Drawing for the job (mm, zero at the part's lowest x, y, z). Give positions to 0.01 mm unless a question says otherwise; leave off trailing zeros. Write each loop counter-clockwise with the first axis right and the second up, starting at its lowest first coordinate (ties: lowest second). Pieces come first, ordered by that corner, then holes.
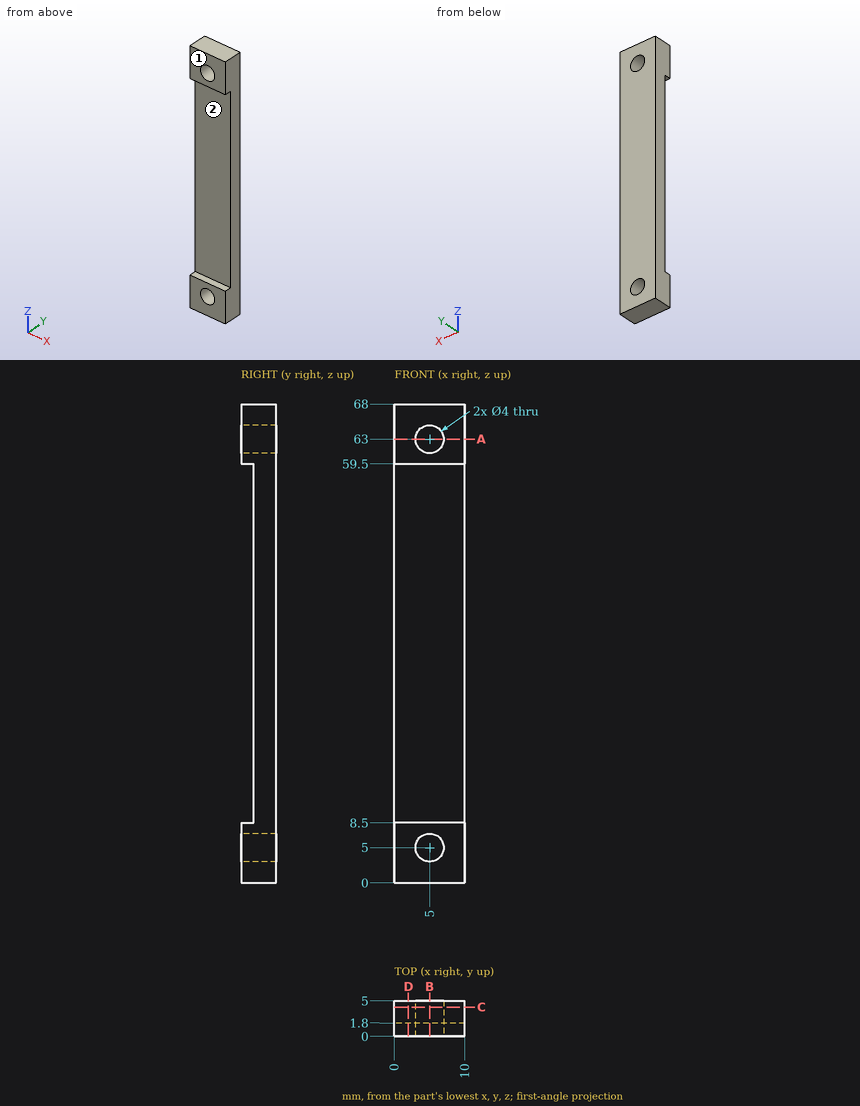
1. Pull direction Z, two halves, no side cores. Call the marked faces 1 and 2: +Z half, -Z half, draft (parallel to the pull), parting line (faces both ways), or undercut.
Calculated:
face 1: draft
face 2: undercut
2. Probe probe 1 along Z at (x, y) = (5, 1.4); probe 2 along Z at (x, y) = (8, 0.2); probe 3 along Z at (x, y) = (5.5, 3.75). List the from-to ranges inside material, lowest first.
Calculated:
probe 1: z = 0 to 3, 7 to 8.5, 59.5 to 61, 65 to 68
probe 2: z = 0 to 8.5, 59.5 to 68
probe 3: z = 0 to 3.06, 6.94 to 61.06, 64.94 to 68
3. Slice it at C-C, the plane y = 4.1. Write the cut outline in (x, z), and give its area (3 significant figures).
Calculated:
outline: (0, 0) - (10, 0) - (10, 68) - (0, 68) - close; hole circle Ø4 at (5, 5); hole circle Ø4 at (5, 63)
area: 655 mm2
4. Slice it at B-B, the plane x = 5. Write the cut outline in (y, z), and give its area (3 significant figures).
Calculated:
outline: (0, 0) - (5, 0) - (5, 3) - (0, 3) - close; (0, 7) - (5, 7) - (5, 61) - (0, 61) - (0, 59.5) - (1.8, 59.5) - (1.8, 8.5) - (0, 8.5) - close; (0, 65) - (5, 65) - (5, 68) - (0, 68) - close
area: 208 mm2
5. Slice it at D-D, the plane x = 2. Write the cut outline in (y, z), and give its area (3 significant figures).
Calculated:
outline: (0, 0) - (5, 0) - (5, 68) - (0, 68) - (0, 59.5) - (1.8, 59.5) - (1.8, 8.5) - (0, 8.5) - close
area: 248 mm2
6. Slice it at A-A, the plane z = 63. Write the cut outline in (x, y).
Calculated:
outline: (0, 0) - (3, 0) - (3, 5) - (0, 5) - close; (7, 0) - (10, 0) - (10, 5) - (7, 5) - close
7. Pin check, flat tip, straight feed: P1, Ø1.5, axis at x = 6, z = 11, coming from the -Y side. Stop position of the tip, or through.
Calculated:
P1: stops at y = 1.8
